The model under review builds one solid part; all positions refer to its coordinate system, in mm. A direction names the side the tool comes from. Coordinates: 2 decimals unless noted, no trailing zeros. Write each loop counter-clockwise with the first axis right and the second up, starting at its lowest first coordinate (ties: lowest second). Pieces come first, ordered by that corner, then holes. Notation, with made-up numbers: (-37.5, -28.5) -> (8.5, -28.5) arc R18 ccw to (8.5, -22.5) -> close; hole circle Ø1 at (-19.75, 60.25). An arc over 180 degrees is marked (long way). Write each question's results on one line, items separated by ' | '.
```python
from build123d import *

# Parameters (mm, degrees)
F0_W     = 60
F0_H     = 45
F0_R     = 6
F1_DEPTH = 25
F2_R     = 2.75
F3_DEPTH = 45
F2_R_2   = 5
F4_DEPTH = 6.5


with BuildPart() as f1:
    # F0 (on Top) → F1 (new body)
    with BuildSketch(Plane.XY):
        Rectangle(F0_W, F0_H)
        with Locations((0, -9.5)):
            Circle(F0_R, mode=Mode.SUBTRACT)
    extrude(amount=F1_DEPTH)

    # F2 (on face) → F3 (cut)
    with BuildSketch(Plane.XZ.offset(22.5)):
        with Locations((-20, 12.798888)):
            Circle(F2_R)
        with Locations((20, 12.798888)):
            Circle(F2_R)
    extrude(amount=-F3_DEPTH, mode=Mode.SUBTRACT)

    # F2 (on face) → F4 (cut)
    with BuildSketch(Plane.XZ.offset(22.5)):
        with Locations((-20, 12.798888)):
            Circle(F2_R_2)
        with Locations((-20, 12.798888)):
            Circle(F2_R, mode=Mode.SUBTRACT)
        with Locations((20, 12.798888)):
            Circle(F2_R_2)
        with Locations((20, 12.798888)):
            Circle(F2_R, mode=Mode.SUBTRACT)
    extrude(amount=-F4_DEPTH, mode=Mode.SUBTRACT)


solid = f1.part
```
Q1. For line 1 (X direction, y = 7, z = 13); line 2 (Z direction, x = 20, y = -18); line 3 (Z direction, x = 20, y = 6), list the stretches that pass through material, from the lowest coordinate up. Write a range as from..to.
Solution:
line 1: -30..-22.74, -17.26..17.26, 22.74..30 | line 2: 0..7.8, 17.8..25 | line 3: 0..10.05, 15.55..25
Q2. Add section B-B (y = -11). Write out the cut boundary in (x, z), plus the area to 3 significant figures.
Solution:
outline: (-30, 0) -> (-5.81, 0) -> (-5.81, 25) -> (-30, 25) -> close; (5.81, 0) -> (30, 0) -> (30, 25) -> (5.81, 25) -> close; hole circle Ø5.5 at (-20, 12.8); hole circle Ø5.5 at (20, 12.8) | area: 1,160 mm²
Q3. Clearance check with a flat-ended pin moving along its axis: P1, Ø5, axis at x = -20, z = 12, coming from the -Y side. State where the tip first meets the part, or that it passes through.
Solution:
P1: y = -16
Q4. Add section C-C (z = 22.25). Write out the cut boundary in (x, y), plus the area to 3 significant figures.
Solution:
outline: (-30, -22.5) -> (30, -22.5) -> (30, 22.5) -> (-30, 22.5) -> close; hole circle Ø12 at (0, -9.5) | area: 2,590 mm²
Q5. Draft analysis for pull direction X (two halves, no side actions). For faces 1 (the cylindrical face through (17.818, 2.98, 11.126)), 2 (the flat face through (0, -22.5, 12)), 3 (the flat face through (30, 0, 12)), state which applies: pulls with the +X half, pulls with the -X half, needs draft (parallel to the pull), parting line crosses it, or undercut.
Solution:
face 1: undercut | face 2: needs draft | face 3: pulls with the +X half
Q6. Machinability: for faces 4 (the flat face through (22.2, -16, 10.6)), 5 (the flat face through (0, 22.5, 12)), which of the approach directions +Z, -Z, +X, -X, +Y, -Y give a long, thin tool a straight path to every point of the face, cutting with its end or side? Answer none if there is none.
Solution:
face 4: -Y | face 5: +Z, -Z, +X, -X, +Y
Q7. Add section A-A (x = 20). Write out the cut boundary in (y, z).
Solution:
outline: (-22.5, 0) -> (22.5, 0) -> (22.5, 10.05) -> (-16, 10.05) -> (-16, 7.8) -> (-22.5, 7.8) -> close; (-22.5, 17.8) -> (-16, 17.8) -> (-16, 15.55) -> (22.5, 15.55) -> (22.5, 25) -> (-22.5, 25) -> close
Q8. Add section D-D (z = 10.75). Write out the cut boundary in (x, y), plus the area to 3 significant figures.
Solution:
outline: (-30, -22.5) -> (-24.56, -22.5) -> (-24.56, -16) -> (-21.83, -16) -> (-21.83, 22.5) -> (-30, 22.5) -> close; (-18.17, -16) -> (-15.44, -16) -> (-15.44, -22.5) -> (15.44, -22.5) -> (15.44, -16) -> (18.17, -16) -> (18.17, 22.5) -> (-18.17, 22.5) -> close; (21.83, -16) -> (24.56, -16) -> (24.56, -22.5) -> (30, -22.5) -> (30, 22.5) -> (21.83, 22.5) -> close; hole circle Ø12 at (0, -9.5) | area: 2,190 mm²
